Check sheet for the modelled part. Datum: model origin and axes. Units: mm. Round coordinates to 2 decimals unless told otherwise and drop trailing zeros. Write each loop counter-clockwise with the first axis right and the second up, starting at its lowest first coordinate (ties: lowest second). Pieces come first, ordered by that corner, then holes.
Item 1: Cross-section at D-D on x = 0. Enter the section's corners in (y, z).
Item 2: Go/stop test with flat-tipped pins: pin 1 Ø8 at (x, z) = (6, 5) entering from +Y; pin 2 Ø6 at (x, z) = (24.5, -2.5) entering from -Y; pin 3 Ø1.6 at (x, z) = (18, -12) entering from +Y. Record where each tip stops, or that it passes through.
Item 3: Release check for a two-part mould opening along Z. For faces 1 (the flat face through (0, -7, 0)), 2 (the cylindrical face through (-1.5, -4.46, 0.07)), 3 (the cylindrical face through (-18.737, -1.014, -11.324)) record: +Z half, -Z half, draft (parallel to the pull), parting line (faces both ways), or undercut.
Item 4: Cross-section at A-A on x = 18. Enter the section's corners in (y, z), plus the area to 3 significant figures.
Item 5: Cross-section at C-C on z = 0. Enter the section's corners in (x, y).
Item 6: Material ranges on line 1 (Z direction, x = 18, y = -1.2); line 2 (Y direction, x = -27, z = -3); line 3 (Z direction, x = -1, y = -4), recorded low to high.
Item 7: Cross-section at B-B on z = 12. Enter the section's corners in (x, y), plus the area to 3 significant figures.
from build123d import *

# Parameters (mm, degrees)
F0_W     = 43
F0_H     = 31
F1_DEPTH = 2
F2_R     = 1.5
F3_DEPTH = 5
F4_R     = 1
F5_DEPTH = 2.001
F6_W     = 43
F6_H     = 31
F6_R     = 1
F6_W_2   = 10
F7_DEPTH = 2
F8_DEPTH = 2.001


with BuildPart() as f1:
    # F0 (on Front) → F1 (new body)
    with BuildSketch(Plane.XZ):
        Rectangle(F0_W, F0_H)
    extrude(amount=F1_DEPTH)

    # F2 (on face) → F3 (join)
    with BuildSketch(Plane.XZ.offset(2)):
        Circle(F2_R)
    extrude(amount=F3_DEPTH)

    # F4 (on face) → F5 (cut, through all)
    with BuildSketch(Plane.XZ.offset(2)):
        with Locations((18, 12)):
            Circle(F4_R)
        with Locations((18, -12)):
            Circle(F4_R)
        with Locations((-18, 12)):
            Circle(F4_R)
        with Locations((-18, -12)):
            Circle(F4_R)
    extrude(amount=-F5_DEPTH, mode=Mode.SUBTRACT)

    # F6 (on Front) → F7 (join)
    with BuildSketch(Plane.XZ):
        Rectangle(F6_W, F6_H)
        with Locations((18, 12)):
            Circle(F6_R, mode=Mode.SUBTRACT)
        with Locations((-26.5, 0)):
            Rectangle(F6_W_2, F6_H)
        with Locations((-26.5, -12)):
            Circle(F6_R, mode=Mode.SUBTRACT)
        with Locations((-26.5, 12)):
            Circle(F6_R, mode=Mode.SUBTRACT)
        with Locations((26.5, 0)):
            Rectangle(F6_W_2, F6_H)
        with Locations((26.5, -12)):
            Circle(F6_R, mode=Mode.SUBTRACT)
        with Locations((26.5, 12)):
            Circle(F6_R, mode=Mode.SUBTRACT)
    extrude(amount=F7_DEPTH)

    # F4 (on face) → F8 (cut, through all)
    with BuildSketch(Plane.XZ.offset(2)):
        with Locations((18, 12)):
            Circle(F4_R)
        with Locations((18, -12)):
            Circle(F4_R)
        with Locations((-18, 12)):
            Circle(F4_R)
        with Locations((-18, -12)):
            Circle(F4_R)
    extrude(amount=-F8_DEPTH, mode=Mode.SUBTRACT)


solid = f1.part
Response values:
1. outline: (-7, -1.5) - (-2, -1.5) - (-2, -15.5) - (0, -15.5) - (0, 15.5) - (-2, 15.5) - (-2, 1.5) - (-7, 1.5) - close
2. pin 1: stops at y = 0
2. pin 2: stops at y = -2
2. pin 3: passes through
3. face 1: draft
3. face 2: parting line
3. face 3: undercut
4. outline: (-2, -15.5) - (0, -15.5) - (0, -13) - (-2, -13) - close; (-2, -11) - (0, -11) - (0, 11) - (-2, 11) - close; (-2, 13) - (0, 13) - (0, 15.5) - (-2, 15.5) - close
4. area: 54.0 mm2
5. outline: (-31.5, -2) - (-1.5, -2) - (-1.5, -7) - (1.5, -7) - (1.5, -2) - (31.5, -2) - (31.5, 0) - (-31.5, 0) - close
6. line 1: z = -15.5 to -13, -11 to 11, 13 to 15.5
6. line 2: y = -2 to 0
6. line 3: z = -1.12 to 1.12
7. outline: (-31.5, -2) - (-27.5, -2) - (-27.5, 0) - (-31.5, 0) - close; (-25.5, -2) - (-19, -2) - (-19, 0) - (-25.5, 0) - close; (-17, -2) - (17, -2) - (17, 0) - (-17, 0) - close; (19, -2) - (25.5, -2) - (25.5, 0) - (19, 0) - close; (27.5, -2) - (31.5, -2) - (31.5, 0) - (27.5, 0) - close
7. area: 110 mm2
